Verification items for the finished model (mm, model axes). Round coordinates to 2 decimals unless told otherwise and drop trailing zeros. Order: outer loops, then holes, each group sorted by start corner. A loop starts at its lowest first (then second) coordinate and runs counter-clockwise, first axis right, second up.
```python
from build123d import *

# Parameters (mm, degrees)
SKETCH006_W     = 14.1
SKETCH006_H     = 14.1
PAD003_DEPTH    = 3
FILLET_R        = 1
CHAMFER001_SIZE = 0.8


with BuildPart() as part:
    # Sketch006 → Pad003 (new body)
    with BuildSketch(Plane.XY):
        Polygon((0, 0), (0, 64.75), (111, 64.75), (111, 27.75), (55.5, 27.75), (55.5, 0), align=None)
        with Locations((27.75, 9.25)):
            Rectangle(SKETCH006_W, SKETCH006_H, mode=Mode.SUBTRACT)
        with Locations((27.75, 55.5)):
            Rectangle(SKETCH006_W, SKETCH006_H, mode=Mode.SUBTRACT)
        with Locations((27.75, 37)):
            Rectangle(SKETCH006_W, SKETCH006_H, mode=Mode.SUBTRACT)
        with Locations((46.25, 55.5)):
            Rectangle(SKETCH006_W, SKETCH006_H, mode=Mode.SUBTRACT)
        with Locations((64.75, 55.5)):
            Rectangle(SKETCH006_W, SKETCH006_H, mode=Mode.SUBTRACT)
        with Locations((83.25, 55.5)):
            Rectangle(SKETCH006_W, SKETCH006_H, mode=Mode.SUBTRACT)
        with Locations((101.75, 55.5)):
            Rectangle(SKETCH006_W, SKETCH006_H, mode=Mode.SUBTRACT)
        with Locations((101.75, 37)):
            Rectangle(SKETCH006_W, SKETCH006_H, mode=Mode.SUBTRACT)
        with Locations((83.25, 37)):
            Rectangle(SKETCH006_W, SKETCH006_H, mode=Mode.SUBTRACT)
        with Locations((64.75, 37)):
            Rectangle(SKETCH006_W, SKETCH006_H, mode=Mode.SUBTRACT)
        with Locations((46.25, 37)):
            Rectangle(SKETCH006_W, SKETCH006_H, mode=Mode.SUBTRACT)
        with Locations((9.25, 55.5)):
            Rectangle(SKETCH006_W, SKETCH006_H, mode=Mode.SUBTRACT)
        with Locations((9.25, 37)):
            Rectangle(SKETCH006_W, SKETCH006_H, mode=Mode.SUBTRACT)
        with Locations((9.25, 9.25)):
            Rectangle(SKETCH006_W, SKETCH006_H, mode=Mode.SUBTRACT)
        with Locations((46.25, 9.25)):
            Rectangle(SKETCH006_W, SKETCH006_H, mode=Mode.SUBTRACT)
    extrude(amount=PAD003_DEPTH)

    # Fillet
    fillet_edges = [part.edges().sort_by_distance(p)[0] for p in [
        (55.5, 0, 1.5),
        (55.5, 27.75, 1.5),
        (111, 27.75, 1.5),
        (0, 0, 1.5),
        (0, 64.75, 1.5),
        (111, 64.75, 1.5),
    ]]
    fillet(fillet_edges, radius=FILLET_R)

    # Chamfer001
    chamfer001_edges = [part.edges().sort_by_distance(p)[0] for p in [
        (83.25, 27.75, 0),
    ]]
    chamfer(chamfer001_edges, length=CHAMFER001_SIZE)


with BuildPart() as part_1:
    # Body002 placement: moved
    add(part.part.moved(Location((18, 0.5, 6.6))))


solid = part_1.part
```
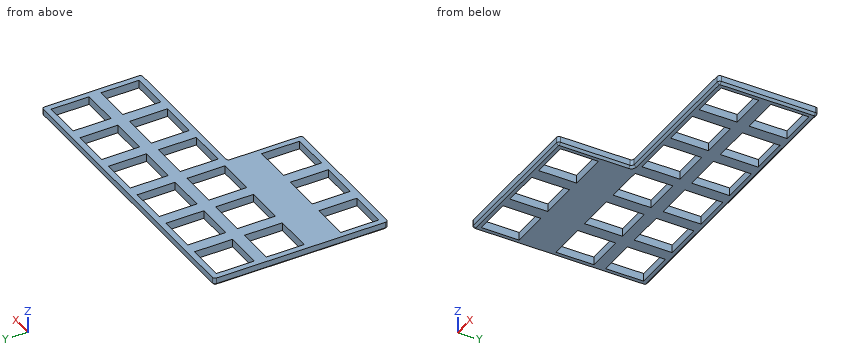
1) Sectioned sample at A-A on y = 41.5. Count the separate pieces of the cut face and the enclosed holes in it, then the cut area to 3 significant figures.
2) Scan lines: probe 1 along Y at (x, z) = (98, 9.4); probe 2 along X at (y, z) = (7, 7.6); probe 3 along Y at (x, z) = (50, 8.65). Record each from-to range of solid material in increasing order.
3) Sectioned sample at D-D on x = 65. Record the cut outline in (y, z), then the cut area to 3 significant figures.
4) Sectioned sample at B-B on x = 87. Record the cut outline in (y, z).
5) Sectioned sample at C-C on y = 13. Record the cut outline in (x, z), then the cut area to 3 significant figures.
Returned:
1. separate pieces: 7
1. enclosed holes: 0
1. area: 78.6 mm2
2. probe 1: y = 28.25 to 30.45, 44.55 to 48.95, 63.05 to 65.25
2. probe 2: x = 18 to 20.2, 34.3 to 38.7, 52.8 to 57.2, 71.3 to 73.5
2. probe 3: y = 0.5 to 2.7, 16.8 to 30.45, 44.55 to 48.95, 63.05 to 65.25
3. outline: (0.5, 7.4) - (1.3, 6.6) - (2.7, 6.6) - (2.7, 9.6) - (0.5, 9.6) - close; (16.8, 6.6) - (30.45, 6.6) - (30.45, 9.6) - (16.8, 9.6) - close; (44.55, 6.6) - (48.95, 6.6) - (48.95, 9.6) - (44.55, 9.6) - close; (63.05, 6.6) - (64.45, 6.6) - (65.25, 7.4) - (65.25, 9.6) - (63.05, 9.6) - close
3. area: 66.7 mm2
4. outline: (28.25, 7.4) - (29.05, 6.6) - (30.45, 6.6) - (30.45, 9.6) - (28.25, 9.6) - close; (44.55, 6.6) - (48.95, 6.6) - (48.95, 9.6) - (44.55, 9.6) - close; (63.05, 6.6) - (64.45, 6.6) - (65.25, 7.4) - (65.25, 9.6) - (63.05, 9.6) - close
5. outline: (18, 7.4) - (18.8, 6.6) - (20.2, 6.6) - (20.2, 9.6) - (18, 9.6) - close; (34.3, 6.6) - (38.7, 6.6) - (38.7, 9.6) - (34.3, 9.6) - close; (52.8, 6.6) - (57.2, 6.6) - (57.2, 9.6) - (52.8, 9.6) - close; (71.3, 6.6) - (72.7, 6.6) - (73.5, 7.4) - (73.5, 9.6) - (71.3, 9.6) - close
5. area: 39.0 mm2
